from build123d import *

# Parameters (mm, degrees)
BOSS_EXTRUDE1_DEPTH = 36.322
CUT_EXTRUDE1_REACH  = 61.511
SKETCH2_R           = 4.572
SKETCH2_W           = 6.096
SKETCH2_H           = 19.2532
BOSS_EXTRUDE2_DEPTH = 1.778
CUT_EXTRUDE2_REACH  = 50.379
SKETCH3_R           = 6.858
SKETCH4_R           = 4.69
SKETCH4_R_2         = 2.15
BOSS_EXTRUDE3_DEPTH = 6
FILLET1_R           = 2.54
CUT_EXTRUDE3_REACH  = 53.279
SKETCH5_W           = 5.588
SKETCH5_H           = 10.16
FILLET2_R           = 1.778
SKETCH6_W           = 1.778
SKETCH6_H           = 0.5
CUT_EXTRUDE4_DEPTH  = 36.322


with BuildPart() as part:
    # Sketch1 → Boss-Extrude1 (new body)
    with BuildSketch(Plane.XY):
        with BuildLine():
            Line((-11.304, 21.082), (11.304, 21.082))
            ThreePointArc((11.304, 21.082), (18.218090106, 18.218090106), (21.082, 11.304))
            Line((21.082, 11.304), (21.082, -11.304))
            ThreePointArc((21.082, -11.304), (18.218090106, -18.218090106), (11.304, -21.082))
            Line((11.304, -21.082), (-11.304, -21.082))
            ThreePointArc((-11.304, -21.082), (-18.218090106, -18.218090106), (-21.082, -11.304))
            Line((-21.082, -11.304), (-21.082, 11.304))
            ThreePointArc((-21.082, 11.304), (-18.218090106, 18.218090106), (-11.304, 21.082))
        make_face()
        with BuildLine():
            Line((-11.304, -19.304), (11.304, -19.304))
            ThreePointArc((11.304, -19.304), (16.960854249, -16.960854249), (19.304, -11.304))
            Line((19.304, -11.304), (19.304, 11.304))
            ThreePointArc((19.304, 11.304), (16.960854249, 16.960854249), (11.304, 19.304))
            Line((11.304, 19.304), (-11.304, 19.304))
            ThreePointArc((-11.304, 19.304), (-16.960854249, 16.960854249), (-19.304, 11.304))
            Line((-19.304, 11.304), (-19.304, -11.304))
            ThreePointArc((-19.304, -11.304), (-16.960854249, -16.960854249), (-11.304, -19.304))
        make_face(mode=Mode.SUBTRACT)
    extrude(amount=BOSS_EXTRUDE1_DEPTH)

    # Sketch2 → Cut-Extrude1 (cut, up to next)
    with BuildSketch(Plane.ZY.offset(21.082), mode=Mode.PRIVATE) as cut_extrude1_sk1:
        with Locations(Location((18.161, 0, 0), (0, 0, 270))):
            Circle(SKETCH2_R)
    cut_extrude1_tool1 = extrude(cut_extrude1_sk1.sketch, amount=-CUT_EXTRUDE1_REACH, mode=Mode.PRIVATE) & part.part
    # Sketch2 → Cut-Extrude1 (cut, up to next)
    with BuildSketch(Plane.ZY.offset(21.082), mode=Mode.PRIVATE) as cut_extrude1_sk2:
        with Locations((8.636, 0)):
            Rectangle(SKETCH2_W, SKETCH2_H)
    cut_extrude1_tool2 = extrude(cut_extrude1_sk2.sketch, amount=-CUT_EXTRUDE1_REACH, mode=Mode.PRIVATE) & part.part
    add(cut_extrude1_tool1.solids().sort_by_distance((-21.082, 0, 18.161))[0], mode=Mode.SUBTRACT)
    add(cut_extrude1_tool2.solids().sort_by_distance((-21.082, 0, 8.636))[0], mode=Mode.SUBTRACT)

    # Sketch1<2> → Boss-Extrude2 (add)
    with BuildSketch(Plane.XY):
        with BuildLine():
            ThreePointArc((-21.082, 11.304), (-18.218090106, 18.218090106), (-11.304, 21.082))
            Line((-11.304, 21.082), (11.304, 21.082))
            ThreePointArc((11.304, 21.082), (18.218090106, 18.218090106), (21.082, 11.304))
            Line((21.082, 11.304), (21.082, -11.304))
            ThreePointArc((21.082, -11.304), (18.218090106, -18.218090106), (11.304, -21.082))
            Line((11.304, -21.082), (-11.304, -21.082))
            ThreePointArc((-11.304, -21.082), (-18.218090106, -18.218090106), (-21.082, -11.304))
            Line((-21.082, -11.304), (-21.082, 11.304))
        make_face()
        with BuildLine():
            Line((-19.304, -11.304), (-19.304, 11.304))
            ThreePointArc((-19.304, 11.304), (-16.960854249, 16.960854249), (-11.304, 19.304))
            Line((-11.304, 19.304), (11.304, 19.304))
            ThreePointArc((11.304, 19.304), (16.960854249, 16.960854249), (19.304, 11.304))
            Line((19.304, 11.304), (19.304, -11.304))
            ThreePointArc((19.304, -11.304), (16.960854249, -16.960854249), (11.304, -19.304))
            Line((11.304, -19.304), (-11.304, -19.304))
            ThreePointArc((-11.304, -19.304), (-16.960854249, -16.960854249), (-19.304, -11.304))
        make_face(mode=Mode.SUBTRACT)
        with BuildLine():
            ThreePointArc((-19.304, 11.304), (-16.960854249, 16.960854249), (-11.304, 19.304))
            Line((-11.304, 19.304), (11.304, 19.304))
            ThreePointArc((11.304, 19.304), (16.960854249, 16.960854249), (19.304, 11.304))
            Line((19.304, 11.304), (19.304, -11.304))
            ThreePointArc((19.304, -11.304), (16.960854249, -16.960854249), (11.304, -19.304))
            Line((11.304, -19.304), (-11.304, -19.304))
            ThreePointArc((-11.304, -19.304), (-16.960854249, -16.960854249), (-19.304, -11.304))
            Line((-19.304, -11.304), (-19.304, 11.304))
        make_face()
    extrude(amount=-BOSS_EXTRUDE2_DEPTH)

    # Sketch3 → Cut-Extrude2 (cut, up to next)
    with BuildSketch(Plane(origin=(0, 0, -1.778), x_dir=(-1, 0, 0), z_dir=(0, 0, -1)), mode=Mode.PRIVATE) as cut_extrude2_sk1:
        Circle(SKETCH3_R)
    cut_extrude2_tool1 = extrude(cut_extrude2_sk1.sketch, amount=-CUT_EXTRUDE2_REACH, mode=Mode.PRIVATE) & part.part
    add(cut_extrude2_tool1.solids().sort_by_distance((0, 0, -1.778))[0], mode=Mode.SUBTRACT)

    # Sketch4 → Boss-Extrude3 (add)
    with BuildSketch(Plane(origin=(0, 21.082, 0), x_dir=(1, 0, 0), z_dir=(0, 1, 0))):
        with Locations(Location((0, -17.272, 0), (0, 0, 90))):
            Circle(SKETCH4_R)
        with Locations(Location((0, -17.272, 0), (0, 0, 270))):
            Circle(SKETCH4_R_2, mode=Mode.SUBTRACT)
    boss_extrude3 = extrude(amount=BOSS_EXTRUDE3_DEPTH)

    # Mirror1: Boss-Extrude3 across plane
    add(boss_extrude3.mirror(Plane.ZX))

    # Fillet1
    fillet1_edges = [part.edges().sort_by_distance(p)[0] for p in [
        (0, 21.082, 21.962),
        (0, -21.082, 21.962),
    ]]
    fillet(fillet1_edges, radius=FILLET1_R)

    # Sketch5 → Cut-Extrude3 (cut, up to next)
    with BuildSketch(Plane(origin=(0, 0, -1.778), x_dir=(-1, 0, 0), z_dir=(0, 0, -1)), mode=Mode.PRIVATE) as cut_extrude3_sk1:
        with Locations((-16.51, 0)):
            Rectangle(SKETCH5_W, SKETCH5_H)
    cut_extrude3_tool1 = extrude(cut_extrude3_sk1.sketch, amount=-CUT_EXTRUDE3_REACH, mode=Mode.PRIVATE) & part.part
    add(cut_extrude3_tool1.solids().sort_by_distance((16.51, 0, -1.778))[0], mode=Mode.SUBTRACT)

    # Fillet2
    fillet2_edges = [part.edges().sort_by_distance(p)[0] for p in [
        (13.716, 5.08, -0.889),
        (13.716, -5.08, -0.889),
    ]]
    fillet(fillet2_edges, radius=FILLET2_R)

    # Sketch6 → Cut-Extrude4 (cut)
    with BuildSketch(Plane.XY.offset(36.322)):
        with Locations((20.193, 0)):
            Rectangle(SKETCH6_W, SKETCH6_H)
    extrude(amount=-CUT_EXTRUDE4_DEPTH, mode=Mode.SUBTRACT)


solid = part.part
Verification items for the finished model (mm, model axes). A direction names the side the tool comes from. Round coordinates to 2 decimals unless told otherwise and drop trailing zeros. Loops run counter-clockwise (first coordinate to the right, second up) from the corner with the lowest first, then second, coordinate; pieces in that order, holes last. Notation, with made-up numbers: M 87,-38 L 146,-38 A33 ccw 146,-3 Z; hole C 76,3.5 d5. An arc over 180 degrees is marked long. Write each question's results on one line, items separated by ' | '.
1) Access from +Z, -Z, +X, -X, +Y, -Y to the whole of each face (thin tool, end or side, straight path). Record for faces 1 (the cylindrical face through (-16.9, 17.02, 17.91)), 2 (the cylindrical face through (0.095, 24.04, 15.124)), 3 (the flat face through (17, 5.08, -1)), 4 (the flat face through (20, -0.25, 18)), 5 (the flat face through (-20, 0, 11.684)).
Checks:
face 1: +Z | face 2: +Y | face 3: +Z, -Z | face 4: +Z, +X | face 5: -X
2) Gauge pin test, flat ends, axial feed: P1, Ø4.5, axis at x = -0.5, z = 16.5, coming from the +Y side; P2, Ø0.9, axis at x = 17, z = -0.5, coming from the +Y side; P3, Ø8, axis at x = -3.5, y = -9.5, coming from the +Z side; P4, Ø3.5, axis at x = 0, z = 17.272, coming from the -Y side. Record the tip position at first contact, or that the pin passes through.
Checks:
P1: stops at y = 27.08 | P2: stops at y = 19.56 | P3: stops at z = 0 | P4: stops at y = -21.08
3) Mould release check, pull along X, two halves, no side actions. Record for faces 6 (the flat face through (-20, -9.627, 9)), 7 (the cylindrical face through (-1.41, -25.33, 12.8)), 8 (the flat face through (17, -5.08, -1)): released by +X, released by -X, zero draft, split by the parting line, or undercut.
Checks:
face 6: zero draft | face 7: split by the parting line | face 8: undercut
4) Section check C-C on x = 12.5. Record the boundary of the cut face in (y, z), then the cut area to 3 significant figures.
Checks:
outline: M -21.01,-1.78 L 21.01,-1.78 L 21.01,36.32 L 19.21,36.32 L 19.21,0 L -19.21,0 L -19.21,36.32 L -21.01,36.32 Z | area: 205 mm2
5) Section check A-A on z = 30.5. Record the boundary of the cut face in (x, y), then the cut area to 3 significant figures.
Checks:
outline: M -21.08,-11.3 A9.78 ccw -11.3,-21.08 L 11.3,-21.08 A9.78 ccw 21.08,-11.3 L 21.08,-0.25 L 19.3,-0.25 L 19.3,-11.3 A8 cw 11.3,-19.3 L -11.3,-19.3 A8 cw -19.3,-11.3 L -19.3,11.3 A8 cw -11.3,19.3 L 11.3,19.3 A8 cw 19.3,11.3 L 19.3,0.25 L 21.08,0.25 L 21.08,11.3 A9.78 ccw 11.3,21.08 L -11.3,21.08 A9.78 ccw -21.08,11.3 Z | area: 259 mm2
6) Scan lines: L1, parallel to Z at x = -20, y = 0; L2, parallel to Y at x = -6.5, z = 22. Record each from-to range of solid material in increasing order. Write a range as from..to.
Checks:
L1: z = -1.78..5.59, 11.68..13.59, 22.73..36.32 | L2: y = -21.08..-19.3, 19.3..21.08
7) Section check B-B on y = -10.5. Record the boundary of the cut face in (x, z).
Checks:
outline: M -21.08,-1.78 L 21.08,-1.78 L 21.08,36.32 L 19.3,36.32 L 19.3,0 L -19.3,0 L -19.3,36.32 L -21.08,36.32 Z
